```python
from build123d import *

# Parameters (mm, degrees)
REVOLVE2_ANGLE     = 360
CUT_EXTRUDE2_DEPTH = 1.54
SKETCH6_R          = 1.443375673
CUT_EXTRUDE3_DEPTH = 1.54
CUT_EXTRUDE3_DRAFT = -45


with BuildPart() as part:
    # Sketch10 → Revolve3 (revolve)
    with BuildSketch(Plane(origin=(0, 0, 0), x_dir=(0, 0, -1), z_dir=(1, 0, 0))):
        Polygon((8.475, 2), (9, 1.475), (9, 0), (-9, 0), (-9, 2), align=None)
    revolve(axis=Axis((0, 0, 11.2), (0, 0, -1)))

    # Sketch7 → Revolve2 (revolve, symmetric)
    with BuildSketch(Plane(origin=(0, 0, 0), x_dir=(0, 0, -1), z_dir=(1, 0, 0))) as revolve2_sk:
        with BuildLine():
            Line((-9.33, 3.8), (-9, 3.8))
            Line((-9, 3.8), (-9, 0))
            Line((-9, 0), (-11.2, 0))
            Line((-11.2, 0), (-11.2, 2))
            ThreePointArc((-11.2, 2), (-10.406499853, 3.047002626), (-9.33, 3.8))
        make_face()
    revolve(axis=Axis((0, 0, 11.2), (0, 0, -1)), revolution_arc=REVOLVE2_ANGLE / 2)
    revolve(revolve2_sk.sketch, axis=Axis((0, 0, 11.2), (0, 0, 1)), revolution_arc=REVOLVE2_ANGLE / 2)

    # Sketch5 → Cut-Extrude2 (cut)
    with BuildSketch(Plane.XY.offset(11.2)):
        Polygon((1.25, -0.721687836), (1.25, 0.721687836), (0, 1.443375673), (-1.25, 0.721687836), (-1.25, -0.721687836), (0, -1.443375673), align=None)
    extrude(amount=-CUT_EXTRUDE2_DEPTH, mode=Mode.SUBTRACT)


with BuildPart() as cut_extrude3_tool:
    # Sketch6 → Cut-Extrude3 (with draft: the straight prism first)
    with BuildSketch(Plane.XY.offset(11.2)):
        Circle(SKETCH6_R)
    extrude(amount=-CUT_EXTRUDE3_DEPTH)
    # Cut-Extrude3: the draft: its side faces are tilted about the plane it starts from
    cut_extrude3_sides = [cut_extrude3_tool.faces().sort_by_distance(p)[0] for p in [
        (-1.443375673, 0, 10.43),
    ]]
    draft(cut_extrude3_sides, Plane.XY.offset(11.2), CUT_EXTRUDE3_DRAFT)


with BuildPart() as part_1:
    add(part.part)

    # Cut-Extrude3: cut by cut_extrude3_tool
    add(cut_extrude3_tool.part, mode=Mode.SUBTRACT)


solid = part_1.part
```
Work out the finished part from the listing and answer in its coordinate system (mm). A direction names the side the tool comes from. Give positions to 0.01 mm unless a question says otherwise; leave off trailing zeros. Write each loop counter-clockwise with the first axis right and the second up, starting at its lowest first coordinate (ties: lowest second). Pieces come first, ordered by that corner, then holes. Notation, with made-up numbers: (69, 46.5) -> (84, 46.5) arc R35 cw to (84, 81.5) -> close; hole circle Ø2 at (31.25, 69). An arc over 180 degrees is marked (long way). Write each question's results on one line, items separated by ' | '.
1. Find section B-B on z = -5.5. Determine the outline of the cut face in (x, y), and give its area (3 significant figures).
Data:
outline: circle Ø4 at (0, 0) | area: 12.6 mm^2
2. Each of these flat-tipped pins is pushed along its axis until it touches: pin 1 Ø1 at (x, y) = (-0.5, 2.5) entering from +Z; pin 2 Ø1.5 at (x, y) = (-2.5, 1.5) entering from +Z; pin 3 Ø1.6 at (y, z) = (0, 10.5) entering from -X. Where does it stop, or does it pass through?
Data:
pin 1: z = 11.17 | pin 2: z = 11.11 | pin 3: x = -3.6
3. Find section C-C on x = 2.25. Determine the outline of the cut face in (y, z).
Data:
outline: (-3.06, 9) -> (3.06, 9) -> (3.06, 9.33) arc R3.58 ccw to (-3.06, 9.33) -> close
4. Straight lines are drawn through the part: L1, parallel to Z at x = -0.75, y = -0.25; L2, parallel to X at y = -0.75, z = 10; L3, parallel to Y at x = 0, z = 3.75. For each, find the intervals that lie inside material, in ascending order.
Data:
L1: -9 to 9.66 | L2: -3.31 to -1.2, 1.2 to 3.31 | L3: -2 to 2
5. Find section A-A on y = 0. Determine the outline of the cut face in (x, z) (3 decimals), and give its area (3 significant figures).
Data:
outline: (-3.8, 9) -> (-2, 9) -> (-2, -8.475) -> (-1.475, -9) -> (1.475, -9) -> (2, -8.475) -> (2, 9) -> (3.8, 9) -> (3.8, 9.33) arc R4.229 ccw to (2, 11.2) -> (1.443, 11.2) -> (1.25, 11.007) -> (1.25, 9.66) -> (-1.25, 9.66) -> (-1.25, 11.007) -> (-1.443, 11.2) -> (-2, 11.2) arc R4.229 ccw to (-3.8, 9.33) -> close | area: 81.9 mm^2
6. Determine the mould class of faces 3 (the cylindrical face through (-2, 0, 0)), 4 (the flat face through (-0.63, -1.08, 10.44)), 5 (the flat face through (2, 2, 9)) for opening direction X: +X half, -X half, draft (parallel to the pull), parting line (faces both ways), or undercut.
Data:
face 3: parting line | face 4: undercut | face 5: draft
7. A tool of negligible diameter and unlimited length cuts with its end or side. For faces 1 (the flat face through (0.616, -1.088, 10.441)), 2 (the cylindrical face through (-0.167, -3.796, 9.163)), from which of +Z, -Z, +X, -X, +Y, -Y can it reach the whole face along a straight path? Write none if from no direction.
Data:
face 1: +Z | face 2: +Z, -Z
8. Find section D-D on x = -2.75. Determine the outline of the cut face in (y, z), and give its area (3 significant figures).
Data:
outline: (-2.62, 9) -> (2.62, 9) -> (2.62, 9.33) arc R3.21 ccw to (-2.62, 9.33) -> close | area: 6.72 mm^2
